Part model, mm, in its own coordinate system. Round coordinates to 2 decimals unless told otherwise and drop trailing zeros. Order: outer loops, then holes, each group sorted by start corner. A loop starts at its lowest first (then second) coordinate and runs counter-clockwise, first axis right, second up. Notation, with made-up numbers: (84.25, 88.5) -> (88.25, 88.5) arc R20 ccw to (88.25, 95.5) -> close; hole circle Ø5 at (46.25, -4). An arc over 180 degrees is marked (long way). Use CSV: the item, a comma, the result in double quotes.
```python
from build123d import *

# Parameters (mm, degrees)
F0_W   = 152.4
F0_H   = 76.2
F0_W_2 = 127


with BuildPart() as f1:
    # F0 (on Top) → F1 (revolve)
    with BuildSketch(Plane.XY):
        with Locations((-214.321307, 102.507023)):
            Rectangle(F0_W, F0_H)
        Polygon((-138.121307, 64.407023), (0, 0), (0, 76.2), (-138.121307, 140.607023), align=None)
        with Locations((63.5, 38.1)):
            Rectangle(F0_W_2, F0_H)
    revolve(axis=Axis((127, 38.1, 0), (0, 1, 0)))


solid = f1.part
```
(1) Cut at C-C, the plane y = 102.5. Give the cut face in (x, z).
Reply:
outline,"circle Ø835.04 at (127, 0); hole circle Ø366.8 at (127, 0)"
(2) Pull direction Z, two halves, no side cores. Call faces 1 (the face through (-146, 64.407, 6)), 2 (the face through (129, 76.2, 2)), 3 (the face through (458.331, 103.04, -254.055)): released by +Z, released by -Z, zero draft, split by the parting line, or undercut.
Reply:
face 1,"zero draft"
face 2,"undercut"
face 3,"split by the parting line"
(3) Cut at D-D, the plane y = 17.5. Give the cut face in (x, z).
Reply:
outline,"circle Ø329.06 at (127, 0)"
(4) Cut at A-A, the plane x = 127. Give the cut face in (y, z), then the cut area to 3 significant figures.
Reply:
outline,"(0, -127) -> (64.41, -265.12) -> (64.41, -417.52) -> (140.61, -417.52) -> (140.61, -265.12) -> (76.2, -127) -> (76.2, 127) -> (140.61, 265.12) -> (140.61, 417.52) -> (64.41, 417.52) -> (64.41, 265.12) -> (0, 127) -> close"
area,"63,600 mm2"
(5) Probe probe 1 along Y at (x, z) = (330, -351.5); probe 2 along Z at (x, y) = (106, 89.5); probe 3 along X at (y, z) = (97, -5.5). List the from-to ranges inside material, lowest first. Write a range as [from, to].
Reply:
probe 1,"[64.41, 140.61]"
probe 2,"[-416.99, -154.1], [154.1, 416.99]"
probe 3,"[-290.49, -44.52], [298.52, 544.49]"
(6) Drop flat-ended pins along their axis: P1, Ø2, axis at x = 242, y = 88, coming from the -Z side; P2, Ø4, axis at x = 332.5, z = -22.5, coming from the -Y side; P3, Ø5, axis at x = 180.5, y = 19.5, coming from the -Z side. Give the stop position or say it passes through.
Reply:
P1,"z = -401.66"
P2,"y = 36.25"
P3,"z = -165.82"
(7) Cut at B-B, the plane z = 0. Give the cut face in (x, y), then the cut area to 3 significant figures.
Reply:
outline,"(-290.52, 64.41) -> (-138.12, 64.41) -> (0, 0) -> (254, 0) -> (392.12, 64.41) -> (544.52, 64.41) -> (544.52, 140.61) -> (392.12, 140.61) -> (254, 76.2) -> (0, 76.2) -> (-138.12, 140.61) -> (-290.52, 140.61) -> close"
area,"63,600 mm2"
